Work out the finished part from the listing and answer in its coordinate system (mm). A direction names the side the tool comes from. Coordinates: 2 decimals unless noted, no trailing zeros. Write each loop counter-clockwise with the first axis right and the second up, starting at its lowest first coordinate (ties: lowest second). Pieces come first, ordered by that corner, then holes. Notation, with made-up numbers: (56.5, 39) - (86.5, 39) arc R12 ccw to (86.5, 53) - close; hole circle Ø6 at (-20.75, 78.25). An arc over 180 degrees is marked (long way). Use one line per item in the form item = value. Start each with the question number.
Item 1: Consider probe 1 along X at (y, z) = (2.05, 7.5); probe 2 along X at (y, z) = (15.75, 13); probe 3 along X at (y, z) = (3.8, 7.5). Determine where each line is inside the solid, lowest interval first.
Item 2: Determine the mould class of faces 1 (the cylindrical face through (-63.43, 24.4, 7.4)), 2 (the cylindrical face through (-78.43, 1.52, 0.6)), 3 (the flat face through (-29, 21, 15)), 4 (the cylindrical face through (14.352, 2.535, 6.026)) for opening direction Z: released by +Z, released by -Z, zero draft, split by the parting line, or undercut.
Item 3: Given pin 1 (4 mm diameter, centred on x = 13.5, z = 8, fed in from +Y); pin 2 (4.5 mm diameter, centred on y = 14.5, z = 6, fed in from +X); pin 3 (4 mm diameter, centred on x = -66.5, y = 13.5, fed in from -Z) (1 decimal); pin 4 (1.5 mm diameter, centred on y = 18.5, z = 8.5, fed in from -X), each flat-ended and moving along its own axis, determine where each tip first touches the part or whether it passes through.
Item 4: A cutting plane is placed at A-A (y = 15.25). Write down the section's boundary in (x, z), then the cut area to 3 significant figures.
Item 5: A cutting plane is placed at B-B (z = 7.5). Write down the section's boundary in (x, y), then the cut area to 3 significant figures.
Item 6: A cutting plane is placed at C-C (x = 13). Write down the section's boundary in (y, z), then the cut area to 3 significant figures.
Item 7: A cutting plane is placed at D-D (x = -26.5). Write down the section's boundary in (y, z), then the cut area to 3 significant figures.
Item 8: For faces 5 (the cylindrical face through (-72.94, 4.43, 0.6)), 6 (the flat face through (11, 5, 9)), 7 (the flat face through (-75, 5, 9)), determine the directions among +Z, -Z, +X, -X, +Y, -Y from which every point of the face is accessible in a straight line to the end or side of a thin tool.
from build123d import *

# Parameters (mm, degrees)
SKETCH1_W           = 15
SKETCH1_H           = 15
SKETCH1_W_2         = 4
SKETCH1_W_3         = 60
BOSS_EXTRUDE1_DEPTH = 25
SKETCH1_3_W         = 60
SKETCH1_3_H         = 15
CUT_EXTRUDE1_DEPTH  = 20
CUT_EXTRUDE2_START  = 25
SKETCH1_4_W         = 15
SKETCH1_4_H         = 15
CUT_EXTRUDE2_DEPTH  = 20
FILLET1_R           = 2
FILLET2_R           = 2
FILLET3_R           = 5
CUT_EXTRUDE3_REACH  = 84.861
SKETCH2_R           = 2


with BuildPart() as part:
    # Sketch1 → Boss-Extrude1 (new body)
    with BuildSketch(Plane(origin=(0, 0, 0), x_dir=(1, 0, 0), z_dir=(0, 1, 0))):
        with Locations((-71.5, -7.5)):
            Rectangle(SKETCH1_W, SKETCH1_H)
        with Locations((-62, -7.5)):
            Rectangle(SKETCH1_W_2, SKETCH1_H)
        with Locations((-30, -7.5)):
            Rectangle(SKETCH1_W_3, SKETCH1_H)
        with Locations((2, -7.5)):
            Rectangle(SKETCH1_W_2, SKETCH1_H)
        with Locations((11.5, -7.5)):
            Rectangle(SKETCH1_W, SKETCH1_H)
    extrude(amount=BOSS_EXTRUDE1_DEPTH)

    # Sketch1<3> → Cut-Extrude1 (cut)
    with BuildSketch(Plane(origin=(0, 0, 0), x_dir=(1, 0, 0), z_dir=(0, 1, 0))):
        with Locations((-30, -7.5)):
            Rectangle(SKETCH1_3_W, SKETCH1_3_H)
    extrude(amount=CUT_EXTRUDE1_DEPTH, mode=Mode.SUBTRACT)

    # Sketch1<4> → Cut-Extrude2 (cut)
    with BuildSketch(Plane(origin=(0, 0, 0), x_dir=(1, 0, 0), z_dir=(0, 1, 0)).offset(CUT_EXTRUDE2_START)):
        with Locations((-71.5, -7.5)):
            Rectangle(SKETCH1_4_W, SKETCH1_4_H)
        with Locations((11.5, -7.5)):
            Rectangle(SKETCH1_4_W, SKETCH1_4_H)
    extrude(amount=-CUT_EXTRUDE2_DEPTH, mode=Mode.SUBTRACT)

    # Fillet1
    fillet1_edges = [part.edges().sort_by_distance(p)[0] for p in [
        (19, 2.5, 0),
        (19, 2.5, 15),
        (-79, 2.5, 15),
        (-79, 2.5, 0),
        (-64, 25, 7.5),
        (4, 25, 7.5),
    ]]
    fillet(fillet1_edges, radius=FILLET1_R)

    # Fillet2
    fillet2_edges = [part.edges().sort_by_distance(p)[0] for p in [
        (-70.5, 5, 0),
        (-70.5, 5, 15),
        (10.5, 5, 15),
        (10.5, 5, 0),
        (19, 5, 7.5),
        (18.414213562, 5, 14.414213562),
        (18.414213562, 5, 0.585786438),
        (-79, 5, 7.5),
        (-78.414213562, 5, 14.414213562),
        (-78.414213562, 5, 0.585786438),
    ]]
    fillet(fillet2_edges, radius=FILLET2_R)

    # Fillet3
    # the kernel refuses this fillet: 5 mm, written as the material it adds along each edge
    with BuildSketch(Plane(origin=(-64, 5, 13), x_dir=(-1, 0, 0), z_dir=(0, 0, -1))) as fillet3_piece_1:
        with BuildLine():
            CenterArc((FILLET3_R, FILLET3_R), FILLET3_R, 180, 90)
            Line((0, FILLET3_R), (0, 0))
            Line((0, 0), (FILLET3_R, 0))
        make_face()
    extrude(amount=11)
    with BuildSketch(Plane(origin=(4, 5, 13), x_dir=(1, 0, 0), z_dir=(0, 0, -1))) as fillet3_piece_2:
        with BuildLine():
            CenterArc((FILLET3_R, -FILLET3_R), FILLET3_R, 90, 90)
            Line((0, -FILLET3_R), (0, 0))
            Line((0, 0), (FILLET3_R, 0))
        make_face()
    extrude(amount=11)
    with BuildSketch(Plane(origin=(-64, 3, 13), x_dir=(0, 0.9999802608561372, -0.00628314396555929), z_dir=(0, 0.00628314396555929, 0.9999802608561372))) as fillet3_piece_3_section:
        with BuildLine():
            CenterArc((-2 - FILLET3_R, FILLET3_R), FILLET3_R, 270, 90)
            Line((-2 - FILLET3_R, 0), (-2, 0))
            Line((-2, 0), (-2, FILLET3_R))
        make_face()
    fillet3_piece_3 = revolve(axis=Axis((-64, 3, 13), (-1, 0, 0)), revolution_arc=359.64, mode=Mode.PRIVATE)
    fillet3_piece_3 = split(fillet3_piece_3, bisect_by=Plane(origin=(-65.84257052, 4.524977571, 15), z_dir=(0, 0, -1)), keep=Keep.TOP, mode=Mode.PRIVATE)
    fillet3_piece_3 = split(fillet3_piece_3, bisect_by=Plane(origin=(-65.84257052, 0, 14.524977571), z_dir=(0, 1, 0)), keep=Keep.TOP, mode=Mode.PRIVATE)
    add(fillet3_piece_3)
    with BuildSketch(Plane(origin=(4, 3, 13), x_dir=(0, 1, 0), z_dir=(0, 0, -1))) as fillet3_piece_4_section:
        with BuildLine():
            CenterArc((2 + FILLET3_R, FILLET3_R), FILLET3_R, 180, 90)
            Line((2 + FILLET3_R, 0), (2, 0))
            Line((2, 0), (2, FILLET3_R))
        make_face()
    fillet3_piece_4 = revolve(axis=Axis((4, 3, 13), (1, 0, 0)), revolution_arc=359.64, mode=Mode.PRIVATE)
    fillet3_piece_4 = split(fillet3_piece_4, bisect_by=Plane(origin=(5.842570594, 4.524977559, 15), z_dir=(0, 0, -1)), keep=Keep.TOP, mode=Mode.PRIVATE)
    fillet3_piece_4 = split(fillet3_piece_4, bisect_by=Plane(origin=(5.842570594, 0, 14.524977563), z_dir=(0, 1, 0)), keep=Keep.TOP, mode=Mode.PRIVATE)
    add(fillet3_piece_4)
    with BuildSketch(Plane(origin=(-64, 3, 2), x_dir=(0, 0.9999802608561372, 0.006283143965558735), z_dir=(0, 0.006283143965558735, -0.9999802608561372))) as fillet3_piece_5_section:
        with BuildLine():
            CenterArc((-2 - FILLET3_R, -FILLET3_R), FILLET3_R, 0, 90)
            Line((-2 - FILLET3_R, 0), (-2, 0))
            Line((-2, 0), (-2, -FILLET3_R))
        make_face()
    fillet3_piece_5 = revolve(axis=Axis((-64, 3, 2), (1, 0, 0)), revolution_arc=359.64, mode=Mode.PRIVATE)
    fillet3_piece_5 = split(fillet3_piece_5, bisect_by=Plane(origin=(-65.842570484, 4.524977652, 0), z_dir=(0, 0, 1)), keep=Keep.TOP, mode=Mode.PRIVATE)
    fillet3_piece_5 = split(fillet3_piece_5, bisect_by=Plane(origin=(-65.842570484, 0, 0.47502245), z_dir=(0, 1, 0)), keep=Keep.TOP, mode=Mode.PRIVATE)
    add(fillet3_piece_5)
    with BuildSketch(Plane(origin=(4, 3, 2), x_dir=(0, 1, 0), z_dir=(0, 0, 1))) as fillet3_piece_6_section:
        with BuildLine():
            CenterArc((2 + FILLET3_R, -FILLET3_R), FILLET3_R, 90, 90)
            Line((2, -FILLET3_R), (2, 0))
            Line((2, 0), (2 + FILLET3_R, 0))
        make_face()
    fillet3_piece_6 = revolve(axis=Axis((4, 3, 2), (-1, 0, 0)), revolution_arc=359.64, mode=Mode.PRIVATE)
    fillet3_piece_6 = split(fillet3_piece_6, bisect_by=Plane(origin=(4.944030812, 6.137069115, 0), z_dir=(0, 0, 1)), keep=Keep.TOP, mode=Mode.PRIVATE)
    fillet3_piece_6 = split(fillet3_piece_6, bisect_by=Plane(origin=(4.944030812, 0, 1.077199574), z_dir=(0, 1, 0)), keep=Keep.TOP, mode=Mode.PRIVATE)
    add(fillet3_piece_6)

    # Sketch2 → Cut-Extrude3 (cut, up to next)
    with BuildSketch(Plane(origin=(0, 5, 0), x_dir=(1, 0, 0), z_dir=(0, 1, 0)), mode=Mode.PRIVATE) as cut_extrude3_sk1:
        with Locations(Location((13, -7.5, 0), (0, 0, 270))):
            Circle(SKETCH2_R)
    cut_extrude3_tool1 = extrude(cut_extrude3_sk1.sketch, amount=-CUT_EXTRUDE3_REACH, mode=Mode.PRIVATE) & part.part
    # Sketch2 → Cut-Extrude3 (cut, up to next)
    with BuildSketch(Plane(origin=(0, 5, 0), x_dir=(1, 0, 0), z_dir=(0, 1, 0)), mode=Mode.PRIVATE) as cut_extrude3_sk2:
        with Locations(Location((-73, -7.5, 0), (0, 0, 270))):
            Circle(SKETCH2_R)
    cut_extrude3_tool2 = extrude(cut_extrude3_sk2.sketch, amount=-CUT_EXTRUDE3_REACH, mode=Mode.PRIVATE) & part.part
    add(cut_extrude3_tool1.solids().sort_by_distance((13, 5, 7.5))[0], mode=Mode.SUBTRACT)
    add(cut_extrude3_tool2.solids().sort_by_distance((-73, 5, 7.5))[0], mode=Mode.SUBTRACT)


solid = part.part
Answer:
q1.probe_1 = -79 to -75, -71 to -60, 0 to 11, 15 to 19
q1.probe_2 = -64 to -60, 0 to 4
q1.probe_3 = -78.83 to -75, -71 to -60, 0 to 11, 15 to 18.83
q2.face_1 = zero draft
q2.face_2 = released by -Z
q2.face_3 = released by +Z
q2.face_4 = undercut
q3.pin_1 = 5
q3.pin_2 = 4
q3.pin_3 = through
q3.pin_4 = -64
q4.outline = (-64, 0) - (-60, 0) - (-60, 15) - (-64, 15) - close; (0, 0) - (4, 0) - (4, 15) - (0, 15) - close
q4.area = 120 mm²
q5.outline = (-79, 0) - (-75, 0) - (-75, 5) - (-77, 5) arc R2 ccw to (-79, 3) - close; (-71, 0) - (-60, 0) - (-60, 20) - (0, 20) - (0, 0) - (11, 0) - (11, 5) - (9, 5) arc R5 cw to (4, 10) - (4, 23) arc R2 ccw to (2, 25) - (-62, 25) arc R2 ccw to (-64, 23) - (-64, 10) arc R5 cw to (-69, 5) - (-71, 5) - close; (15, 0) - (19, 0) - (19, 3) arc R2 ccw to (17, 5) - (15, 5) - close
q5.area = 617 mm²
q6.outline = (0, 0) - (3, 0) arc R2 ccw to (5, 2) - (5, 5.5) - (0, 5.5) - close; (0, 9.5) - (5, 9.5) - (5, 13) arc R2 ccw to (3, 15) - (0, 15) - close
q6.area = 53.3 mm²
q7.outline = (20, 0) - (25, 0) - (25, 15) - (20, 15) - close
q7.area = 75.0 mm²
q8.face_5 = -Z, -X, +Y
q8.face_6 = +Z, -Z, +X, +Y
q8.face_7 = +Z, -Z, -X, +Y
